```python
from build123d import *

# Parameters (mm, degrees)
SIDECONNECTIONCUTOUT_DEPTH      = 73.071040696
SIDECONNECTIONCUTOUT_DEPTH_BACK = 73.071040696


with BuildPart() as part:
    # ProfileS → Profile (revolve)
    with BuildSketch(Plane(origin=(0, 0, 0), x_dir=(1, 0, 0), z_dir=(0, 1, 0))):
        with BuildLine():
            Line((10, 58.044891829), (10.291196376, 33.398198054))
            ThreePointArc((10.291196376, 33.398198054), (11.210065487, 27.929487559), (13.75, 23))
            Line((13.75, 23), (11.555755546, 23))
            ThreePointArc((11.555755546, 23), (9.29389864, 27.974053085), (8.476604376, 33.376758967))
            Line((8.476604376, 33.376758967), (8.185408, 58.023452742))
            ThreePointArc((8.185408, 58.023452742), (6.786696454, 63.308767571), (3.05, 67.299763243))
            Line((3.05, 67.299763243), (3.05, 69.398198054))
            ThreePointArc((3.05, 69.398198054), (8.088410722, 64.678596949), (10, 58.044891829))
        make_face()
    revolve(axis=Axis((0, 0, -23), (0, 0, -1)))

    # SideConnectionCutoutS → SideConnectionCutout (cut, two sides)
    with BuildSketch(Plane(origin=(0, 0, 0), x_dir=(0, 0, -1), z_dir=(1, 0, 0))) as sideconnectioncutout_sk:
        with BuildLine():
            Line((56, -2.75), (49, -2.75))
            ThreePointArc((49, -2.75), (46.25, 0), (49, 2.75))
            Line((49, 2.75), (56, 2.75))
            ThreePointArc((56, 2.75), (58.75, 0), (56, -2.75))
        make_face()
    extrude(amount=SIDECONNECTIONCUTOUT_DEPTH, mode=Mode.SUBTRACT)
    extrude(sideconnectioncutout_sk.sketch, amount=-SIDECONNECTIONCUTOUT_DEPTH_BACK, mode=Mode.SUBTRACT)


solid = part.part
```
Could you check a few things on this model? Use its own coordinates, in mm. A direction names the side the tool comes from. Round coordinates to 2 decimals unless told otherwise and drop trailing zeros. Loops run counter-clockwise (first coordinate to the right, second up) from the corner with the lowest first, then second, coordinate; pieces in that order, holes last.
Q1. Please list where these lines run through material, in increasing order: L1, parallel to X at y = 0, z = -67.9; L2, parallel to X at y = 0, z = -68.05; L3, parallel to Y at x = 7, z = -49.
Q2. On a 3-axis mill with a long thin cutter (end or side, diameter ignored), from which of +Z, -Z, +X, -X, +Y, -Y can I reach the whole of each face in a straight line? I mean faces 1 (the conical face through (-1.81, 8.13, -45.87)), 2 (the conical face through (9.374, 3.887, -45.549)), 3 (the cylindrical face through (-8.84, 0.06, -58.75)). Say none if no direction works.
Q3. I want a section at B-B (z = -39). Write out the boundary of the cut face in (x, y), and give its area (3 significant figures).
Q4. I want a section at C-C (y = 0). Give the number of separate pieces and of enclosed holes in the cut face, and give its area (3 significant figures).
Q5. Thinking about a two-plate mould opening in Z: for faces 4 (the flat face through (-3.1, -11.3, -23)), 5 (the flat face through (9, -2.75, -53)), 6 (the cylindrical face through (-3.047, -0.134, -68.364)), which applies, pulls with the +Z half, pulls with the -Z half, needs draft (parallel to the pull), parting line crosses it, or undercut?
Q6. For P1, Ø6, axis at y = -4.5, z = -47, coming from the +X side; P2, Ø1, axis at x = -8.5, z = -51, coming from the -Y side; P3, Ø4, axis at y = 11, z = -34.5, coming from the -X side, each with a flat end and sliding along its axis, tell me the tip position at first contact or that it passes through.
Q7. I want a section at A-A (z = -48). Write out the boundary of the cut face in (x, y).
Answer below:
1. L1: x = -5.3 to -3.05, 3.05 to 5.3
1. L2: x = -5.11 to -3.05, 3.05 to 5.11
1. L3: y = -7.29 to -4.44, 4.44 to 7.29
2. face 1: +Z
2. face 2: -Z
2. face 3: +X, -X
3. outline: circle Ø20.45 at (0, 0); hole circle Ø16.82 at (0, 0)
3. area: 106 mm2
4. separate pieces: 4
4. enclosed holes: 0
4. area: 130 mm2
5. face 4: pulls with the +Z half
5. face 5: undercut
5. face 6: needs draft
6. P1: stops at x = 10.02
6. P2: stops at y = -6.14
6. P3: stops at x = -4.96
7. outline: (-9.79, -2.56) arc R10.12 ccw to (9.79, -2.56) - (7.9, -2.56) arc R8.3 cw to (-7.9, -2.56) - close; (-9.79, 2.56) - (-7.9, 2.56) arc R8.3 cw to (7.9, 2.56) - (9.79, 2.56) arc R10.12 ccw to start
